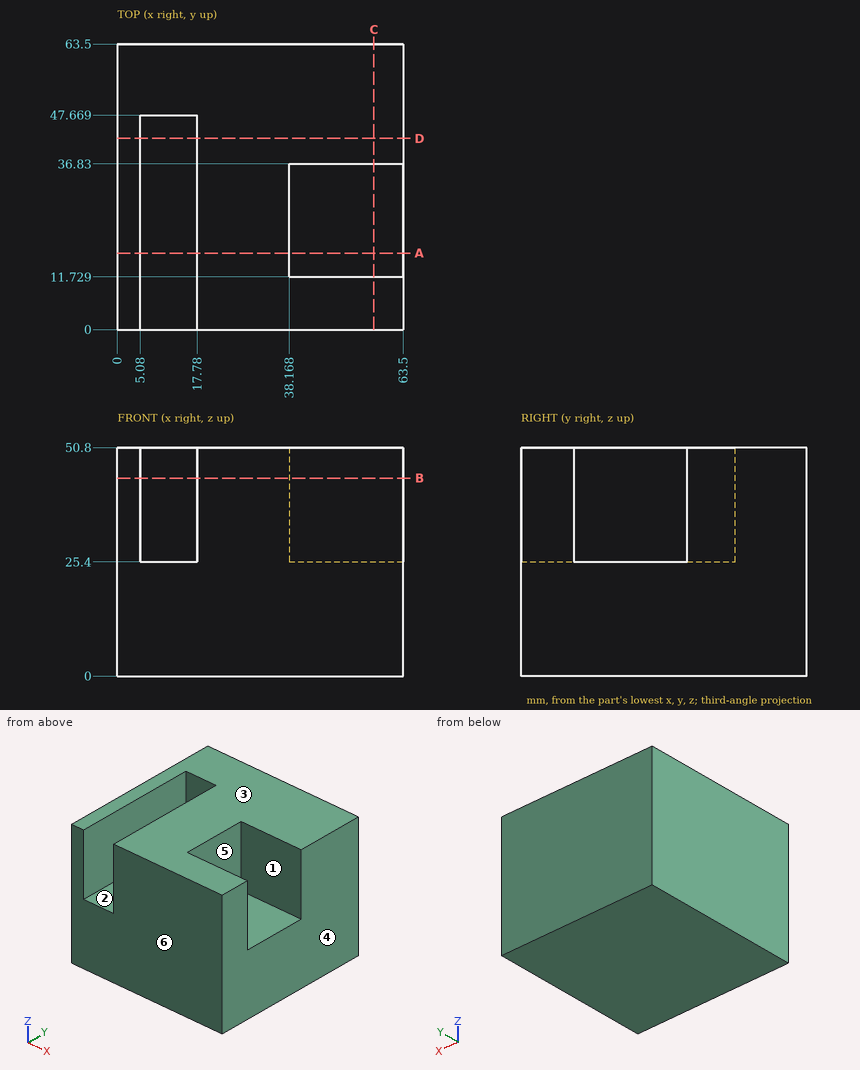
Input: dimensioned drawing with shaded views. Units: mm. Origin: part minimum x, y, z. A direction names the side the tool comes from. Give positions to 0.01 mm unless a question says otherwise; leave off trailing zeros. Order: outer loops, then holes, each group sorted by start corner. A loop starts at its lowest first (then second) coordinate and runs counter-clockwise, first axis right, second up. Notation, with made-up numbers: (47, 7.25) -> (78, 7.25) arc R25 ccw to (78, 36.25) -> close; hole circle Ø2 at (23.25, 63.25). An arc over 180 degrees is marked (long way). Use a Markdown table: item, result.
1) Mould query, pull axis Y, two halves, no side actions, for the marked faces 4, 5 and 6. Classes: +Y half, -Y half, draft (parallel to the pull), parting line (faces both ways), or undercut.
Answer list:
| item | result |
|---|---|
| face 4 | draft |
| face 5 | undercut |
| face 6 | -Y half |
2) Section query C-C, the plane x = 57. Return the cut outline in (y, z), then the cut area to 3 significant figures.
Answer list:
| item | result |
|---|---|
| outline | (0, 0) -> (63.5, 0) -> (63.5, 50.8) -> (36.83, 50.8) -> (36.83, 25.4) -> (11.73, 25.4) -> (11.73, 50.8) -> (0, 50.8) -> close |
| area | 2,590 mm² |
3) Reachability of the marked faces 1, 2 and 3 from +Z, -Z, +X, -X, +Y, -Y: full face, straight path, thin tool, end or side. Return the list, or none.
Answer list:
| item | result |
|---|---|
| face 1 | +Z, +X |
| face 2 | +Z, -Y |
| face 3 | +Z, +X, -X, +Y, -Y |
4) Section query A-A, the plane y = 17. Return the cut outline in (x, z).
Answer list:
| item | result |
|---|---|
| outline | (0, 0) -> (63.5, 0) -> (63.5, 25.4) -> (38.17, 25.4) -> (38.17, 50.8) -> (17.78, 50.8) -> (17.78, 25.4) -> (5.08, 25.4) -> (5.08, 50.8) -> (0, 50.8) -> close |
5) Section query D-D, the plane y = 42.5. Return the cut outline in (x, z), then the cut area to 3 significant figures.
Answer list:
| item | result |
|---|---|
| outline | (0, 0) -> (63.5, 0) -> (63.5, 50.8) -> (17.78, 50.8) -> (17.78, 25.4) -> (5.08, 25.4) -> (5.08, 50.8) -> (0, 50.8) -> close |
| area | 2,900 mm² |
6) Contact query for flat-ended pins moving along their axis: P1, Ø6, axis at y = 27, z = 39.5, coming from the +X side; P2, Ø6.5, axis at x = 12, y = 17, coming from the +Z side; P3, Ø5, axis at x = 11.5, z = 43, coming from the -Y side. Output: stop coordinate, or through.
Answer list:
| item | result |
|---|---|
| P1 | x = 38.17 |
| P2 | z = 25.4 |
| P3 | y = 47.67 |
7) Ray query, line 1 along Y through (x, z) = (55, 34.5); line 2 along X through (y, z) = (20.5, 48); line 3 along Y through (x, z) = (14, 27). Return the intervals inside material, ascending. Write a range as [from, to].
Answer list:
| item | result |
|---|---|
| line 1 | [0, 11.73], [36.83, 63.5] |
| line 2 | [0, 5.08], [17.78, 38.17] |
| line 3 | [47.67, 63.5] |
8) Section query B-B, the plane z = 44. Return the cut outline in (x, y), then the cut area to 3 significant figures.
Answer list:
| item | result |
|---|---|
| outline | (0, 0) -> (5.08, 0) -> (5.08, 47.67) -> (17.78, 47.67) -> (17.78, 0) -> (63.5, 0) -> (63.5, 11.73) -> (38.17, 11.73) -> (38.17, 36.83) -> (63.5, 36.83) -> (63.5, 63.5) -> (0, 63.5) -> close |
| area | 2,790 mm² |
